from build123d import *

# Parameters (mm, degrees)
BOSS_EXTRUDE1_DEPTH     = 457.2
CUT_EXTRUDE1_DEPTH      = 23.225
CUT_EXTRUDE1_DEPTH_BACK = 4.175


with BuildPart() as part:
    # Sketch1 → Boss-Extrude1 (new body)
    with BuildSketch(Plane.XY):
        Polygon((0, 0), (25.4, 0), (25.4, 3.175), (3.175, 3.175), (3.175, 25.4), (0, 25.4), align=None)
    extrude(amount=BOSS_EXTRUDE1_DEPTH)

    # Sketch2 → Cut-Extrude1 (cut, two sides)
    with BuildSketch(Plane(origin=(0, 3.175, 0), x_dir=(1, 0, 0), z_dir=(0, 1, 0))) as cut_extrude1_sk:
        Polygon((0, 0), (25.4, -25.4), (25.4, 0), align=None)
        Polygon((0, -457.2), (25.4, -431.8), (25.4, -457.2), align=None)
    extrude(amount=CUT_EXTRUDE1_DEPTH, mode=Mode.SUBTRACT)
    extrude(cut_extrude1_sk.sketch, amount=-CUT_EXTRUDE1_DEPTH_BACK, mode=Mode.SUBTRACT)


solid = part.part
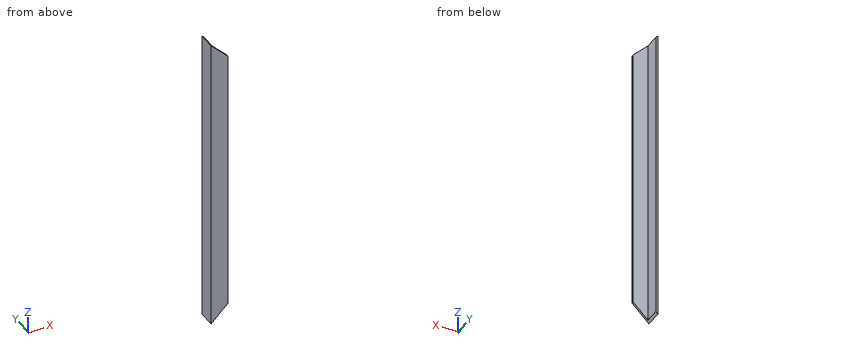
Here's how the part is built. I have some questions about the finished solid (model axes, mm). Coordinates: 2 decimals unless noted, no trailing zeros. Order: outer loops, then holes, each group sorted by start corner. A loop starts at its lowest first (then second) coordinate and runs counter-clockwise, first axis right, second up.
Item 1: If we section it at B-B on x = 18.75: List the corners of the cut face in (y, z) for me (3 decimals), plus the area to 3 significant figures.
Result sheet:
outline: (0, 18.75) - (3.175, 18.75) - (3.175, 438.45) - (0, 438.45) - close
area: 1,330 mm2
Item 2: If we section it at A-A on z = 67: List the corners of the cut face in (x, y) for me (3 decimals).
Result sheet:
outline: (0, 0) - (25.4, 0) - (25.4, 3.175) - (3.175, 3.175) - (3.175, 25.4) - (0, 25.4) - close
Item 3: I need wall thicknesses on line 1 (X direction, y = 8.5, z = 310.5) (3 decimals); line 2 (Z direction, x = 10.25, y = 1.5). Which ranges of each line are inside material? Lowest first, please.
Result sheet:
line 1: x = 0 to 3.175
line 2: z = 10.25 to 446.95
Item 4: If we section it at C-C on y = 7: List the corners of the cut face in (x, z) for me (3 decimals).
Result sheet:
outline: (0, 0) - (3.175, 3.175) - (3.175, 454.025) - (0, 457.2) - close
Item 5: For P1, Ø4, axis at y = 20, z = 246.5, coming from the +X side (3 decimals); P2, Ø11, axis at x = 15.5, z = 226.5, coming from the +Y side (3 decimals); P3, Ø10, axis at x = 5.5, y = 3.5, coming from the -Z side, each with a flat end and sliding along its axis, tell me the tip position at first contact or that it passes through.
Result sheet:
P1: stops at x = 3.175
P2: stops at y = 3.175
P3: stops at z = 0.5
